Check sheet for the modelled part. Datum: model origin and axes. Units: mm. Face numbers are marked on the shaded views. Give positions to 0.01 mm unless a question says otherwise; leave off trailing zeros. Loops run counter-clockwise (first coordinate to the right, second up) from the corner with the lowest first, then second, coordinate; pieces in that order, holes last.
```python
from build123d import *

# Parameters (mm, degrees)
SKETCH1_W               = 40
SKETCH1_H               = 101.6
BOSS_EXTRUDE1_DEPTH     = 49.53
FILLET1_R               = 20
CUT_EXTRUDE2_DEPTH      = 120.899044617
CUT_EXTRUDE2_DEPTH_BACK = 120.899044617
SKETCH2_R               = 7.67


with BuildPart() as part:
    # Sketch1 → Boss-Extrude1 (new body)
    with BuildSketch(Plane.XY):
        with Locations((20, 50.8)):
            Rectangle(SKETCH1_W, SKETCH1_H)
    extrude(amount=BOSS_EXTRUDE1_DEPTH)

    # Fillet1
    fillet1_edges = [part.edges().sort_by_distance(p)[0] for p in [
        (40, 101.6, 24.765),
        (0, 101.6, 24.765),
    ]]
    fillet(fillet1_edges, radius=FILLET1_R - 0.0001)  # a hair under: the kernel refuses the full size

    # Sketch2 → Cut-Extrude2 (cut, two sides: drawn at the far end of the back side and taken through both)
    with BuildSketch(Plane.XY.offset(-CUT_EXTRUDE2_DEPTH_BACK)):
        with Locations((20, 81.6)):
            Circle(SKETCH2_R)
    extrude(amount=CUT_EXTRUDE2_DEPTH + CUT_EXTRUDE2_DEPTH_BACK, mode=Mode.SUBTRACT)


solid = part.part
```
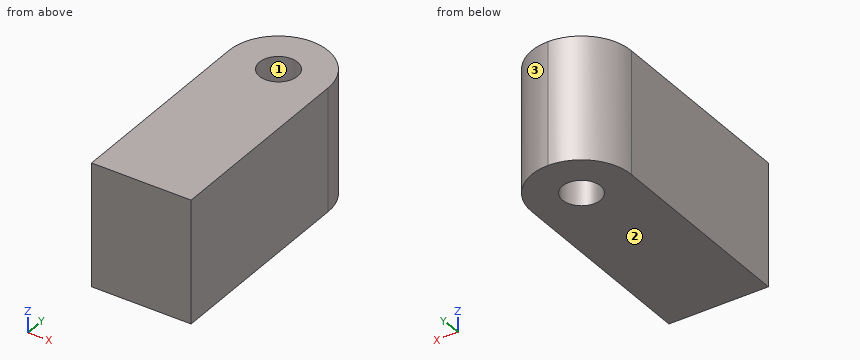
(1) Release check for a two-part mould opening along X. For the marked faces 1, 2 and 3 record: pulls with the +X half, pulls with the -X half, needs draft (parallel to the pull), parting line crosses it, or undercut.
(2) Section check D-D on x = 3. Record the boundary of the cut face in (y, z).
(3) Section check A-A on y = 78. Record the boundary of the cut face in (x, z).
(4) Material ranges on line 1 (Y direction, x = 20, z = 21); line 2 (X direction, y = 81.6, z = 27.5); line 3 (X direction, y = 81, z = 12), recorded low to high.
(5) Gauge pin test, flat ends, axial feed: pin 1 Ø12 at (x, z) = (19, 18.5) entering from -Y; pin 2 Ø1 at (y, z) = (89.5, 19.5) entering from -X; pin 3 Ø8 at (x, z) = (30, 12.5) entering from +Y; pin 4 Ø1 at (x, z) = (10, 28) entering from +Y. Record the tip position at first contact, or that the pin passes through.
(6) Section check C-C on x = 26.5. Record the boundary of the cut face in (y, z), plus the area to 3 significant figures.
Computed values:
1. face 1: undercut
1. face 2: needs draft
1. face 3: pulls with the +X half
2. outline: (0, 0) - (92.14, 0) - (92.14, 49.53) - (0, 49.53) - close
3. outline: (0, 0) - (13.23, 0) - (13.23, 49.53) - (0, 49.53) - close; (26.77, 0) - (40, 0) - (40, 49.53) - (26.77, 49.53) - close
4. line 1: y = 0 to 73.93, 89.27 to 101.6
4. line 2: x = 0 to 12.33, 27.67 to 40
4. line 3: x = 0 to 12.35, 27.65 to 40
5. pin 1: stops at y = 0
5. pin 2: stops at x = 1.42
5. pin 3: stops at y = 100.68
5. pin 4: stops at y = 99.2
6. outline: (0, 0) - (77.53, 0) - (77.53, 49.53) - (0, 49.53) - close; (85.67, 0) - (100.51, 0) - (100.51, 49.53) - (85.67, 49.53) - close
6. area: 4,580 mm2
